Input: dimensioned drawing with shaded views. Units: mm. Origin: part minimum x, y, z. A direction names the side the tool comes from. Give positions to 0.01 mm unless a question says otherwise; leave off trailing zeros. Loops run counter-clockwise (first coordinate to the right, second up) from the corner with the lowest first, then second, coordinate; pieces in that order, holes last. Notation, with made-up numbers: M -1,82 L 27,82 A17 cw 27,105 Z; hole C 76,58.5 d11. An arc over 180 degrees is marked long. Use CSV: the item, a comma, the result in double quotes. Start each with the question number.
Q1. Pull-direction query (X, two-part tool) for the marked faces 1, 2, 3 and 4; classes: released by +X, released by -X, zero draft, split by the parting line, or undercut.
Q2. Section B-B, the plane y = 93. Output: boundary loops of the cut face in (x, z) (1 decimal).
Q3. Reachability of the marked faces 5 and 6 from +Z, -Z, +X, -X, +Y, -Y: full face, straight path, thin tool, end or side. Return the list, or none.
Q4. Section C-C, the plane x = 58. Output: boundary loops of the cut face in (y, z), plus the area to 3 significant figures.
Q5. Section D-D, the plane z = 61. Output: boundary loops of the cut face in (x, y) (1 decimal), plus the area to 3 significant figures.
Q6. Pin query (flat end, axial travel): pin 1 (6 mm diameter, centred on x = 54.5, z = 58.5, fed in from +Y); pin 2 (10 mm diameter, centred on x = 28.1, y = 55.63, fed in from -Z); pin 3 (1 mm diameter, centred on x = 104, z = 8.5, fed in from -Y). Return the tip coordinate at first contact, or that it passes through.
Q7. Section A-A, the plane z = 71.5. Output: boundary loops of the cut face in (x, y) (1 decimal).
Q8. Material intervals for line 1 along Y through (x, z) = (27.5, 18); line 2 along X through (y, z) = (56.5, 41) (1 decimal); line 3 along Y through (x, z) = (113, 41.5), sorted ascending.
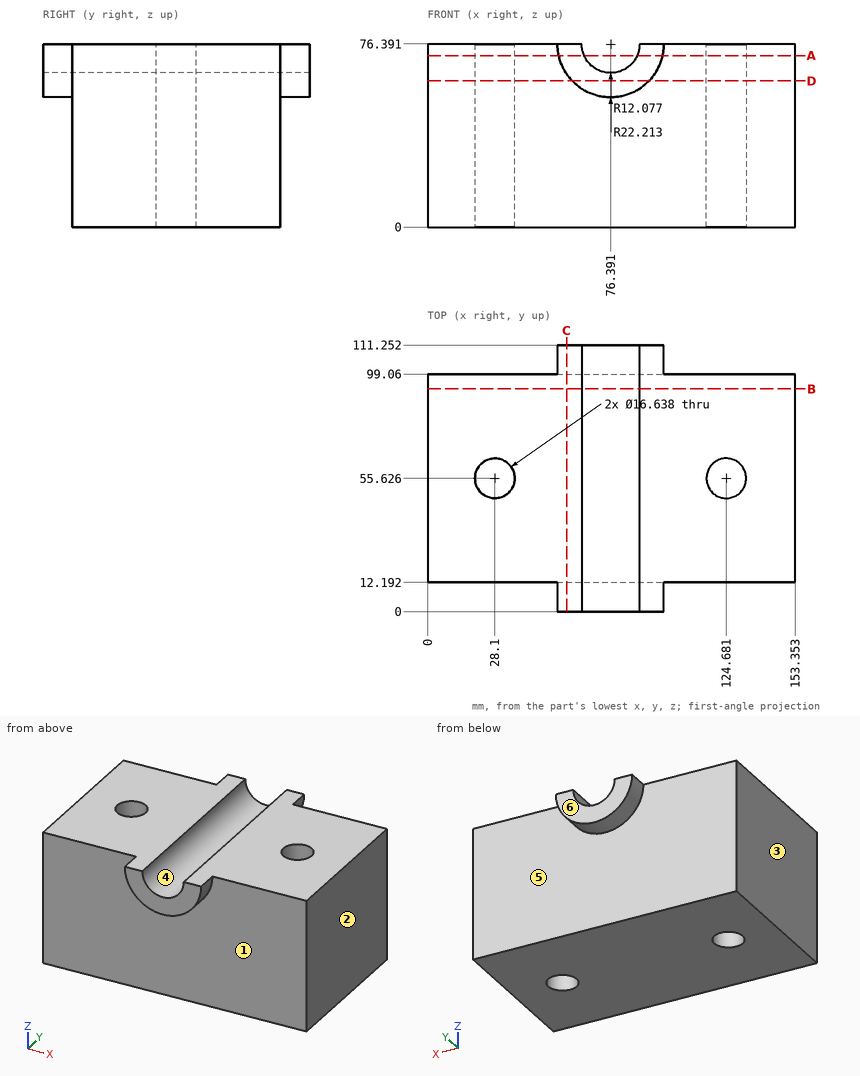
A:
1,face 1,"zero draft"
1,face 2,"released by +X"
1,face 3,"released by -X"
1,face 4,"undercut"
2,outline,"M 0,0 L 153.4,0 L 153.4,76.4 L 88.5,76.4 A12.1 cw 64.3,76.4 L 0,76.4 Z"
3,face 5,"-Z, +Y"
3,face 6,"+Z, -Z, +X, -X, +Y"
4,outline,"M 0,63.93 L 12.19,63.93 L 12.19,0 L 99.06,0 L 99.06,63.93 L 111.25,63.93 L 111.25,76.39 L 0,76.39 Z"
4,area,"6,940 mm^2"
5,outline,"M 0,12.2 L 60.4,12.2 L 60.4,0 L 92.4,0 L 92.4,12.2 L 153.4,12.2 L 153.4,99.1 L 92.4,99.1 L 92.4,111.3 L 60.4,111.3 L 60.4,99.1 L 0,99.1 Z; hole C 28.1,55.6 d16.6; hole C 124.7,55.6 d16.6"
5,area,"13,700 mm^2"
6,pin 1,"y = 99.06"
6,pin 2,"through"
6,pin 3,"y = 12.19"
7,outline,"M 0,12.2 L 54.7,12.2 L 54.7,0 L 65.3,0 L 65.3,111.3 L 54.7,111.3 L 54.7,99.1 L 0,99.1 Z; M 87.4,0 L 98.1,0 L 98.1,12.2 L 153.4,12.2 L 153.4,99.1 L 98.1,99.1 L 98.1,111.3 L 87.4,111.3 Z; hole C 28.1,55.6 d16.6; hole C 124.7,55.6 d16.6"
8,line 1,"12.19 to 47.33, 63.92 to 99.06"
8,line 2,"0 to 19.8, 36.4 to 116.4, 133 to 153.4"
8,line 3,"12.19 to 99.06"
